```python
from build123d import *

# Parameters (mm, degrees)
SKETCH1_R                            = 4.7625
BOSS_EXTRUDE1_DEPTH                  = 254
F_10_24_TAPPED_HOLE1_D               = 3.7973
F_10_24_TAPPED_HOLE1_DEPTH           = 12.83
F_10_24_TAPPED_HOLE1_TIP             = 1.140824014
F_10_24_TAPPED_HOLE1_ON_FACE_2_D     = 3.7973
F_10_24_TAPPED_HOLE1_ON_FACE_2_DEPTH = 12.83
F_10_24_TAPPED_HOLE1_ON_FACE_2_TIP   = 1.140824014


with BuildPart() as part:
    # Sketch1 → Boss-Extrude1 (new body)
    with BuildSketch(Plane(origin=(0, 0, 0), x_dir=(1, 0, 0), z_dir=(0, 1, 0))):
        with Locations(Location((0, 0, 0), (0, 0, 270))):
            Circle(SKETCH1_R)
    extrude(amount=BOSS_EXTRUDE1_DEPTH)

    # #10-24 Tapped Hole1
    with Locations(Plane.ZX.offset(254)):
        with Locations((0, 0)):
            Hole(F_10_24_TAPPED_HOLE1_D / 2, depth=F_10_24_TAPPED_HOLE1_DEPTH)
            with Locations((0, 0, -(F_10_24_TAPPED_HOLE1_DEPTH + F_10_24_TAPPED_HOLE1_TIP / 2))):  # 118° drill point
                Cone(0, F_10_24_TAPPED_HOLE1_D / 2, F_10_24_TAPPED_HOLE1_TIP, mode=Mode.SUBTRACT)

    # #10-24 Tapped Hole1 on face 2
    with Locations(Plane(origin=(0, 0, 0), x_dir=(0, 0, -1), z_dir=(0, -1, 0))):
        with Locations((0, 0)):
            Hole(F_10_24_TAPPED_HOLE1_ON_FACE_2_D / 2, depth=F_10_24_TAPPED_HOLE1_ON_FACE_2_DEPTH)
            with Locations((0, 0, -(F_10_24_TAPPED_HOLE1_ON_FACE_2_DEPTH + F_10_24_TAPPED_HOLE1_ON_FACE_2_TIP / 2))):  # 118° drill point
                Cone(0, F_10_24_TAPPED_HOLE1_ON_FACE_2_D / 2, F_10_24_TAPPED_HOLE1_ON_FACE_2_TIP, mode=Mode.SUBTRACT)


solid = part.part
```
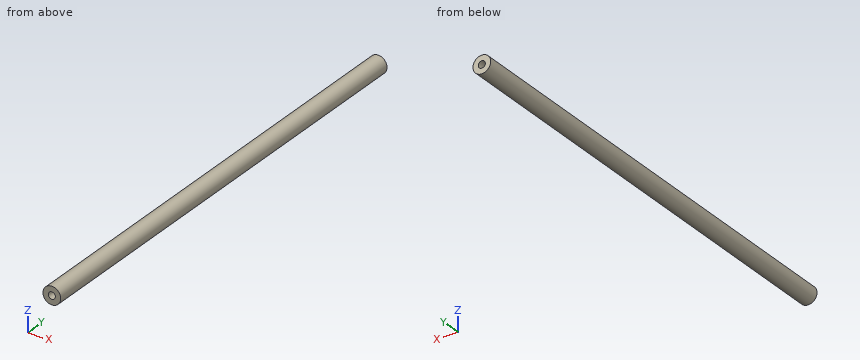
Geometry check sheet. Reference: the model listing, model coordinates, mm. Give positions to 0.01 mm unless a question says otherwise; leave off trailing zeros. Write each loop counter-clockwise with the first axis right and the second up, starting at its lowest first coordinate (ties: lowest second). Pieces come first, ordered by that corner, then holes.
1) Material ranges on L1, parallel to X at y = 4, z = 0; L2, parallel to Z at x = -2.5, y = 91.5; L3, parallel to X at y = 12, z = -2.25, recorded low to high.
2) Section check A-A, the plane y = 212. Record the boundary of the cut face in (x, z) (1 decimal), and give its area (3 significant figures).
3) Gauge pin test, flat ends, axial feed: pin 1 (2.5 mm diameter, centred on x = 0, z = 0, fed in from +Y); pin 2 (5 mm diameter, centred on y = 97.5, z = -3, fed in from -X); pin 3 (1.5 mm diameter, centred on x = 1, y = 209.5, fed in from -Z). Record the tip position at first contact, or that the pin passes through.
Computed:
1. L1: x = -4.76 to -1.9, 1.9 to 4.76
1. L2: z = -4.05 to 4.05
1. L3: x = -4.2 to 4.2
2. outline: circle Ø9.5 at (0, 0)
2. area: 71.3 mm2
3. pin 1: stops at y = 240.78
3. pin 2: stops at x = -4.74
3. pin 3: stops at z = -4.76
